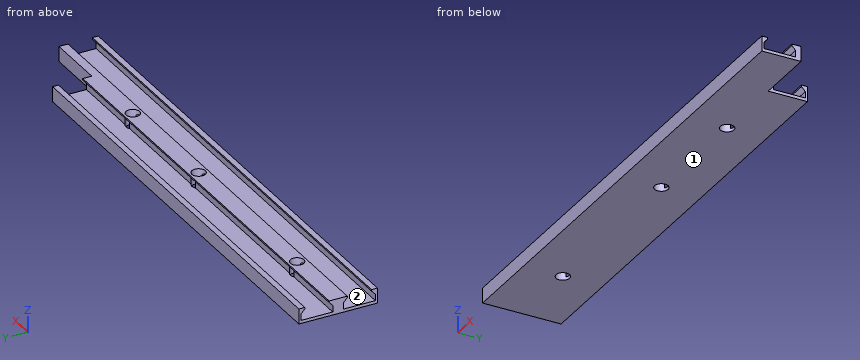
from build123d import *

# Parameters (mm, degrees)
F1_DEPTH = 85
F2_W     = 20
F2_H     = 13
F3_DEPTH = 5.001
F4_R     = 2.25
F5_DEPTH = 5


with BuildPart() as f1:
    # F0 (on Right) → F1 (new body, symmetric)
    with BuildSketch(Plane.YZ):
        Polygon((13, -2.5), (13, 2.5), (11.05, 2.5), (11.05, 1.9975107236), (12.3, 0.6552975509), (12.3, -1.5), (1.8, -1.5), (1.8, 0.7089860778), (3, 1.9975107236), (3, 2.5), (-3, 2.5), (-3, 1.9975107236), (-1.8, 0.7089860778), (-1.8, -1.5), (-12.3, -1.5), (-12.3, 0.6552975509), (-11.05, 1.9975107236), (-11.05, 2.5), (-13, 2.5), (-13, -2.5), align=None)
    extrude(amount=F1_DEPTH, both=True)

    # F2 (on face) → F3 (cut, through all)
    with BuildSketch(Plane(origin=(0, 0, -2.5), x_dir=(1, 0, 0), z_dir=(0, 0, -1))):
        with Locations((75, -6.5)):
            Rectangle(F2_W, F2_H)
    extrude(amount=-F3_DEPTH, mode=Mode.SUBTRACT)

    # F4 (on face) → F5 (cut, through all)
    with BuildSketch(Plane.XY.offset(2.5)):
        with Locations((-60, 0)):
            Circle(F4_R)
        Circle(F4_R)
        with Locations((40, 0)):
            Circle(F4_R)
    extrude(amount=-F5_DEPTH, mode=Mode.SUBTRACT)


solid = f1.part
Part model, mm, in its own coordinate system. Face numbers are marked on the shaded views. Give positions to 0.01 mm unless a question says otherwise; leave off trailing zeros. Order: outer loops, then holes, each group sorted by start corner. A loop starts at its lowest first (then second) coordinate and runs counter-clockwise, first axis right, second up. Notation, with made-up numbers: (-28.75, 58.5) - (28.25, 58.5) arc R9 cw to (28.25, 66.5) - close; hole circle Ø6 at (85.25, -16). An arc over 180 degrees is marked (long way). Use a Markdown table: item, result.
1) Saw through at A-A on x = -9. List the corners of the cut face in (y, z).
Checked values:
| item | result |
|---|---|
| outline | (-13, -2.5) - (13, -2.5) - (13, 2.5) - (11.05, 2.5) - (11.05, 2) - (12.3, 0.66) - (12.3, -1.5) - (1.8, -1.5) - (1.8, 0.71) - (3, 2) - (3, 2.5) - (-3, 2.5) - (-3, 2) - (-1.8, 0.71) - (-1.8, -1.5) - (-12.3, -1.5) - (-12.3, 0.66) - (-11.05, 2) - (-11.05, 2.5) - (-13, 2.5) - close |
2) Two-plate mould, pull along Y, no slides. Class the marked faces 1 and 2: +Y half, -Y half, draft (parallel to the pull), parting line (faces both ways), or undercut.
Checked values:
| item | result |
|---|---|
| face 1 | draft |
| face 2 | undercut |
3) Probe L1, parallel to Y at x = 29.5, z = -0.95; L2, parallel to X at y = 0.5, z = -1.6; L3, parallel to Y at x = 40, z = 0.3. List the from-to ranges inside material, lowest first. Write a range as from..to.
Checked values:
| item | result |
|---|---|
| L1 | -13..-12.3, -1.8..1.8, 12.3..13 |
| L2 | -85..-62.19, -57.81..-2.19, 2.19..37.81, 42.19..65 |
| L3 | -13..-12.3, 12.3..13 |
4) Saw through at C-C on y = 8. List the corners of the cut face in (x, z).
Checked values:
| item | result |
|---|---|
| outline | (-85, -2.5) - (65, -2.5) - (65, -1.5) - (-85, -1.5) - close |
5) Saw through at B-B on y = -5.75. List the corners of the cut face in (x, z).
Checked values:
| item | result |
|---|---|
| outline | (-85, -2.5) - (85, -2.5) - (85, -1.5) - (-85, -1.5) - close |
6) Flat gauge pins, fed straight in: P1, Ø4, axis at x = -60, y = 0, coming from the +Z side; P2, Ø4, axis at x = -7, y = -5.5, coming from the +Z side; P3, Ø2.5, axis at x = 71.5, z = 0.5, coming from the +Y side. Where does each tip first touch, or does it go through?
Checked values:
| item | result |
|---|---|
| P1 | through |
| P2 | z = -1.5 |
| P3 | y = 0 |
